Part model, mm, in its own coordinate system. A direction names the side the tool comes from. Coordinates: 2 decimals unless noted, no trailing zeros. Write each loop counter-clockwise with the first axis right and the second up, starting at its lowest first coordinate (ties: lowest second). Pieces come first, ordered by that corner, then holes. Notation, with made-up numbers: M 65,14.5 L 117,14.5 A17 ccw 117,43.5 Z; hole C 41.5,75 d1. An arc over 180 degrees is marked long. Use a Markdown table: item, result. Add a question column.
Q1. Pin check, flat tips, straight feed: pin 1 Ø4 at (y, z) = (-34.5, 13) entering from +X; pin 2 Ø6 at (x, y) = (130, 16.5) entering from +Z. Stop position of each tip, or through.
Q2. Wall check: L1, parallel to Z at x = 175.45, y = 13.5; L2, parallel to X at y = 26, z = -9; L3, parallel to Y at x = 175.7, z = -27. Give the ranges that are in metal, low to high. Write a range as from..to.
Q3. Slice it at A-A on x = 86. Write the cut outline in (y, z).
Q4. Mould opens along X. For faces 1 (the cylindrical face through (49.3, -0.64, 45.88)), 2 (the flat face through (176, 13, -25)), 3 (the cylindrical face through (175.493, -12.346, -21.165)), 4 (the conical face through (117.255, -0.621, 41.256)) say: released by +X, released by -X, zero draft, split by the parting line, or undercut.
Q5. Slice it at C-C on x = 227.5. Write the cut outline in (y, z), then the cut area to 3 significant figures.
Q6. Tool access for faces 5 (the flat face through (176, 29, 0)), 6 (the flat face through (176, -14, -25)), 7 (the cylindrical face through (175.5, -24.5, 0.1)), 8 (the cylindrical face through (285.49, -1.32, 29.97)): list every direction of +Z, -Z, +X, -X, +Y, -Y with a clear straight run to the whole face (end or side of a thin tool).
Q7. Slice it at B-B on x = 163.5. Write the cut outline in (y, z).
Autodesk Fusion 360 part; units mm, degrees
sketch "Sketch1" plane through (0, 0, 0) normal (1, 0, 0) x (0, 0, -1)
  line L0 (0, 0) -> (0, 45)
  line L1 (0, 0) -> (0, -45)
  line L2 (0, 45) -> (37.5, 45)
  line L3 (0, 45) -> (-37.5, 45)
  line L4 (0, -45) -> (37.5, -45)
  line L5 (0, -45) -> (-37.5, -45)
  arc A0 (-37.5, 45) -> (-37.5, -45) centre (79.119, 0) ccw
  arc A1 (37.5, -45) -> (37.5, 45) centre (-79.119, 0) ccw
  dimension "d1" = 45
  dimension "d2" = 45
  dimension "d3" = 37.5
  dimension "d4" = 37.5
  dimension "d5" = 37.5
  dimension "d6" = 37.5
  dimension "d8" = 125
extrude "Extrude1" add sketch "Sketch1" along normal blind 100
extrude "Extrude2" add 1 faces at (100, -15.2642, -14.2806) along direction (1, 0, 0) blind 35 draft -15
sketch "Sketch2" plane through (135, 0, 0) normal (1, 0, 0) x (0, 0, -1)
  line L0 (-30.8786, -35.6218) -> (30.8786, -35.6218)
  arc A0 (30.8786, -35.6218) -> (30.8786, 35.6218) centre (-79.119, 0) ccw
  line L1 (30.8786, 35.6218) -> (-30.8786, 35.6218)
  arc A1 (-30.8786, 35.6218) -> (-30.8786, -35.6218) centre (79.119, 0) ccw
  circle A2 centre (0, 0) radius 34.5
  dimension "d13" = 69
extrude "Extrude3" add sketch "Sketch2" along normal blind 10 contours A2
sketch "Sketch3" plane through (145, 0, 0) normal (1, 0, 0) x (0, 0, -1)
  circle A0 centre (0, 0) radius 34.5
  circle A1 centre (0, 0) radius 31
  dimension "d16" = 62
extrude "Extrude4" add sketch "Sketch3" along normal blind 30 contours A1
sketch "Sketch4" plane through (175, 0, 0) normal (1, 0, 0) x (0, 0, -1)
  circle A0 centre (0, 0) radius 31
  line L0 (0, 0) -> (27, 0)
  circle A1 centre (27, 0) radius 2.5
  circle A2 centre (27, 0) radius 1.5
  dimension "d19" = 27
  dimension "d20" = 5
  dimension "d21" = -1
extrude "Extrude5" add sketch "Sketch4" along normal blind 1 contours A1
pattern_circular "C-Pattern1" count 12 over 360 about axis through (175, 0, 0) along (1, 0, 0) of "Extrude5"
sketch "Sketch5" plane through (175, 0, 0) normal (1, 0, 0) x (0, 0, -1)
  circle A0 centre (27, 0) radius 2.5
  circle A1 centre (0, 0) radius 31
  circle A2 centre (23.3827, 13.5) radius 2.5
  circle A3 centre (13.5, 23.3827) radius 2.5
  circle A4 centre (0, 27) radius 2.5
  circle A5 centre (-13.5, 23.3827) radius 2.5
  circle A6 centre (-23.3827, 13.5) radius 2.5
  circle A7 centre (-27, 0) radius 2.5
  circle A8 centre (-23.3827, -13.5) radius 2.5
  circle A9 centre (-13.5, -23.3827) radius 2.5
  circle A10 centre (0, -27) radius 2.5
  circle A11 centre (13.5, -23.3827) radius 2.5
  circle A12 centre (23.3827, -13.5) radius 2.5
  line L0 (0, 0) -> (16, 0)
  line L1 (16, 0) -> (16, 17)
  line L2 (16, 0) -> (16, -17)
  line L3 (0, 0) -> (0, -8.0593)
  line L4 (-16, 0) -> (-16, 17)
  line L5 (-16, 0) -> (-16, -17)
  arc A13 (16, 17) -> (-16, 17) centre (0, 1.9003) ccw
  arc A14 (-16, -17) -> (16, -17) centre (0, -1.9003) ccw
  dimension "d26" = 16
  dimension "d27" = 17
  dimension "d28" = 17
  dimension "d29" = 22
extrude "Extrude6" add sketch "Sketch5" along normal blind 100 contours L1 L2 L4 L5 A13 A14
sketch "Sketch6" plane through (275, 0, 0) normal (1, 0, 0) x (0, 0, -1)
  line L0 (-16, 17) -> (-16, -17)
  arc A0 (-16, -17) -> (16, -17) centre (0, -1.9003) ccw
  line L1 (16, -17) -> (16, 17)
  arc A1 (16, 17) -> (-16, 17) centre (0, 1.9003) ccw
  circle A2 centre (0, 0) radius 31
  circle A3 centre (0, 0) radius 30
  dimension "d32" = 62
  dimension "d35" = -1
extrude "Extrude7" add sketch "Sketch6" along normal blind 10 contours L0 A0 L1 A1 | A2 | A3
sketch "Sketch7" plane through (285, 0, 0) normal (1, 0, 0) x (0, 0, -1)
  circle A0 centre (0, 0) radius 31
  circle A1 centre (0, 0) radius 30
  dimension "d36" = -1
extrude "Extrude8" add sketch "Sketch7" along normal blind 1 contours A1
Recorded:
| question | item | result |
|---|---|---|
| 1 | pin 1 | x = 135 |
| 1 | pin 2 | z = 37.58 |
| 2 | L1 | -25.88..-24.88, -21.88..-20.88, -16..16, 20.88..21.88, 24.88..25.88 |
| 2 | L2 | 0..175, 275..286 |
| 2 | L3 | -2.5..-1.5, 1.5..2.5 |
| 3 | outline | M -45,-37.5 A125 ccw 45,-37.5 L 45,37.5 A125 ccw -45,37.5 Z |
| 4 | face 1 | zero draft |
| 4 | face 2 | undercut |
| 4 | face 3 | undercut |
| 4 | face 4 | released by +X |
| 5 | outline | M -17,-16 L 17,-16 A22 ccw 17,16 L -17,16 A22 ccw Z |
| 5 | area | 1,390 mm² |
| 6 | face 5 | +Z, -Z, +Y |
| 6 | face 6 | -Z, +Y, -Y |
| 6 | face 7 | none |
| 6 | face 8 | +X |
| 7 | outline | C 0,0 d62 |
